Autodesk Inventor part; units mm, degrees
ref_plane "YZ Plane" through (0, 0, 0) normal (1, 0, 0) x (0, 1, 0)
ref_plane "XZ Plane" through (0, 0, 0) normal (0, 1, 0) x (-1, 0, 0)
ref_plane "XY Plane" through (0, 0, 0) normal (0, 0, 1) x (1, 0, 0)
sketch "Sketch1" plane through (0, 0, 0) normal (0, 1, 0) x (-1, 0, 0)
  line L0 (3.6662, -6.35) -> (-3.6662, -6.35)
  line L1 (-3.6662, -6.35) -> (-7.3323, 0)
  line L2 (-7.3323, 0) -> (-3.6662, 6.35)
  line L3 (-3.6662, 6.35) -> (3.6662, 6.35)
  line L4 (3.6662, 6.35) -> (7.3323, 0)
  line L5 (7.3323, 0) -> (3.6662, -6.35)
  circle A0 centre (0, 0) radius 1.905
  dimension "d0" = 12.7
  dimension "d6" = 3.81
extrude "Extrusion1" add sketch "Sketch1" against normal blind 41.275
sketch "Sketch2" plane through (0, 0, 0) normal (0, 1, 0) x (1, 0, 0)
  circle A0 centre (0, 0) radius 4.7625
  circle A1 centre (0, 0) radius 1.905
  dimension "d3" = 9.525
extrude "Extrusion2" add sketch "Sketch2" along normal blind 26.9875
properties part number "Roller shaft"
Input: part model. Units: mm. Frame: model coordinates. A direction names the side the tool comes from. Give positions to 0.01 mm unless a question says otherwise; leave off trailing zeros. Loops run counter-clockwise (first coordinate to the right, second up) from the corner with the lowest first, then second, coordinate; pieces in that order, holes last. Notation, with made-up numbers: M 5.25,1.5 L 21.25,1.5 A24 cw 21.25,21.5 Z; hole C 40,72 d3. An arc over 180 degrees is marked long. Use one line per item in the form item = value.
1. Reachability of faces 1 (the face through (-3.78, 13.3, -2.9)), 2 (the face through (-5.525, -20.349, -3.131)) from +Z, -Z, +X, -X, +Y, -Y: full face, straight path, thin tool, end or side. Return the list, or none.
Numbers:
face_1 = +Y
face_2 = -Z, -X, +Y, -Y
2. Section query B-B, the plane y = -10. Return the cut outline in (x, z) (3 decimals), and give its area (3 significant figures).
Numbers:
outline = M -7.332,0 L -3.666,-6.35 L 3.666,-6.35 L 7.332,0 L 3.666,6.35 L -3.666,6.35 Z; hole C 0,0 d3.81
area = 128 mm²
3. Line query: L1, parallel to X at y = 12.75, z = 0 (1 decimal); L2, parallel to Z at x = 0, y = -14 (3 decimals). Output: solid intervals per line, ascending.
Numbers:
L1 = -4.8 to -1.9, 1.9 to 4.8
L2 = -6.35 to -1.905, 1.905 to 6.35
4. First-contact query: pin 1 (2 mm diameter, centred on x = 5, y = -16, fed in from -Z). Flat tip, straight axial feed; report the tip coordinate or a pass-through.
Numbers:
pin_1 = -5.77
5. Section query C-C, the plane z = -3.5. Return the cut outline in (x, y) (1 decimal), and give its area (3 significant figures).
Numbers:
outline = M -5.3,-41.3 L 5.3,-41.3 L 5.3,0 L 3.2,0 L 3.2,27 L -3.2,27 L -3.2,0 L -5.3,0 Z
area = 613 mm²
